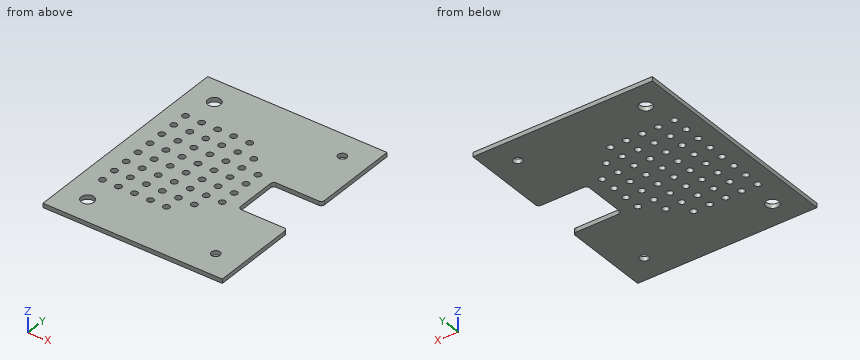
from build123d import *

# Parameters (mm, degrees)
F0_W     = 84
F0_H     = 104
F0_R     = 3
F0_R_2   = 2
F1_DEPTH = 2
F2_W     = 23
F2_H     = 22
F3_DEPTH = 2.001
F4_R     = 1.5
F5_R     = 1.5
F6_DEPTH = 2.001


with BuildPart() as f1:
    # F0 (on Top) → F1 (new body)
    with BuildSketch(Plane.XY):
        Rectangle(F0_W, F0_H)
        with Locations((-30, -40)):
            Circle(F0_R, mode=Mode.SUBTRACT)
        with Locations((30, -40)):
            Circle(F0_R_2, mode=Mode.SUBTRACT)
        with Locations((-30, 40)):
            Circle(F0_R, mode=Mode.SUBTRACT)
        with Locations((30, 40)):
            Circle(F0_R_2, mode=Mode.SUBTRACT)
    extrude(amount=F1_DEPTH)

    # F2 (on face) → F3 (cut, through all)
    with BuildSketch(Plane(origin=(0, 0, 0), x_dir=(1, 0, 0), z_dir=(0, 0, -1))):
        with Locations((30.5, 0)):
            Rectangle(F2_W, F2_H)
    extrude(amount=-F3_DEPTH, mode=Mode.SUBTRACT)

    # F4
    f4_edges = [f1.edges().sort_by_distance(p)[0] for p in [
        (19, 11, 1),
        (42, 11, 1),
        (19, -11, 1),
        (42, -11, 1),
    ]]
    fillet(f4_edges, radius=F4_R)

    # F5 (on face) → F6 (cut, through all)
    with BuildSketch(Plane.XY.offset(2)):
        with Locations((-33.25, -26.25)):
            Circle(F5_R)
        with Locations((-33.25, -18.75)):
            Circle(F5_R)
        with Locations((-33.25, -11.25)):
            Circle(F5_R)
        with Locations((-33.25, -3.75)):
            Circle(F5_R)
        with Locations((-25.75, -26.25)):
            Circle(F5_R)
        with Locations((-25.75, -18.75)):
            Circle(F5_R)
        with Locations((-25.75, -11.25)):
            Circle(F5_R)
        with Locations((-25.75, -3.75)):
            Circle(F5_R)
        with Locations((-18.25, -26.25)):
            Circle(F5_R)
        with Locations((-18.25, -18.75)):
            Circle(F5_R)
        with Locations((-18.25, -11.25)):
            Circle(F5_R)
        with Locations((-18.25, -3.75)):
            Circle(F5_R)
        with Locations((-10.75, -26.25)):
            Circle(F5_R)
        with Locations((-10.75, -18.75)):
            Circle(F5_R)
        with Locations((-10.75, -11.25)):
            Circle(F5_R)
        with Locations((-10.75, -3.75)):
            Circle(F5_R)
        with Locations((-3.25, -26.25)):
            Circle(F5_R)
        with Locations((-3.25, -18.75)):
            Circle(F5_R)
        with Locations((-3.25, -11.25)):
            Circle(F5_R)
        with Locations((-3.25, -3.75)):
            Circle(F5_R)
        with Locations((4.25, -18.75)):
            Circle(F5_R)
        with Locations((4.25, -11.25)):
            Circle(F5_R)
        with Locations((4.25, -3.75)):
            Circle(F5_R)
        with Locations((11.75, -11.25)):
            Circle(F5_R)
        with Locations((11.75, -3.75)):
            Circle(F5_R)
        with Locations((-33.25, 26.25)):
            Circle(F5_R)
        with Locations((-25.75, 26.25)):
            Circle(F5_R)
        with Locations((-25.75, 3.75)):
            Circle(F5_R)
        with Locations((-3.25, 3.75)):
            Circle(F5_R)
        with Locations((-10.75, 26.25)):
            Circle(F5_R)
        with Locations((-3.25, 26.25)):
            Circle(F5_R)
        with Locations((-33.25, 3.75)):
            Circle(F5_R)
        with Locations((-10.75, 3.75)):
            Circle(F5_R)
        with Locations((-33.25, 18.75)):
            Circle(F5_R)
        with Locations((-18.25, 3.75)):
            Circle(F5_R)
        with Locations((-18.25, 18.75)):
            Circle(F5_R)
        with Locations((-25.75, 11.25)):
            Circle(F5_R)
        with Locations((11.75, 11.25)):
            Circle(F5_R)
        with Locations((-25.75, 18.75)):
            Circle(F5_R)
        with Locations((-10.75, 18.75)):
            Circle(F5_R)
        with Locations((-33.25, 11.25)):
            Circle(F5_R)
        with Locations((-3.25, 18.75)):
            Circle(F5_R)
        with Locations((4.25, 18.75)):
            Circle(F5_R)
        with Locations((-10.75, 11.25)):
            Circle(F5_R)
        with Locations((11.75, 3.75)):
            Circle(F5_R)
        with Locations((-18.25, 26.25)):
            Circle(F5_R)
        with Locations((4.25, 3.75)):
            Circle(F5_R)
        with Locations((-3.25, 11.25)):
            Circle(F5_R)
        with Locations((4.25, 11.25)):
            Circle(F5_R)
        with Locations((-18.25, 11.25)):
            Circle(F5_R)
    extrude(amount=-F6_DEPTH, mode=Mode.SUBTRACT)


solid = f1.part
For this review, take the finished solid that the model builds, in its own axes (mm). Round coordinates to 2 decimals unless told otherwise and drop trailing zeros. Order: outer loops, then holes, each group sorted by start corner. A loop starts at its lowest first (then second) coordinate and runs counter-clockwise, first axis right, second up. Notation, with made-up numbers: (-31, 33) -> (0, 33) arc R9 cw to (0, 43) -> close; hole circle Ø10 at (14.25, 0.25). An arc over 180 degrees is marked (long way). Put each result on its own line as item: value.
Q1. For probe 1 along Y at (x, z) = (21, 0.75); probe 2 along Y at (x, z) = (-31.5, 0.8); probe 3 along Y at (x, z) = (-29.5, 1.3), list the stretches that pass through material, from the lowest coordinate up. Write a range as [from, to].
Check result:
probe 1: [-52, -11], [11, 52]
probe 2: [-52, -42.6], [-37.4, 37.4], [42.6, 52]
probe 3: [-52, -42.96], [-37.04, 37.04], [42.96, 52]
Q2. Add section D-D on x = 4.25. Write out the cut boundary in (y, z).
Check result:
outline: (-52, 0) -> (-20.25, 0) -> (-20.25, 2) -> (-52, 2) -> close; (-17.25, 0) -> (-12.75, 0) -> (-12.75, 2) -> (-17.25, 2) -> close; (-9.75, 0) -> (-5.25, 0) -> (-5.25, 2) -> (-9.75, 2) -> close; (-2.25, 0) -> (2.25, 0) -> (2.25, 2) -> (-2.25, 2) -> close; (5.25, 0) -> (9.75, 0) -> (9.75, 2) -> (5.25, 2) -> close; (12.75, 0) -> (17.25, 0) -> (17.25, 2) -> (12.75, 2) -> close; (20.25, 0) -> (52, 0) -> (52, 2) -> (20.25, 2) -> close
Q3. Insertion check: pin 1 Ø5 at (x, y) = (-25.75, 18.75) entering from +Z. The pin has a flat end and moves straight along its axis. Give the tip position at first contact, or say it passes through.
Check result:
pin 1: z = 2
Q4. Add section B-B on x = 25.5. Write out the cut boundary in (y, z), plus the area to 3 significant figures.
Check result:
outline: (-52, 0) -> (-11, 0) -> (-11, 2) -> (-52, 2) -> close; (11, 0) -> (52, 0) -> (52, 2) -> (11, 2) -> close
area: 164 mm2
Q5. Add section C-C on y = -3.75. State how many separate pieces and enclosed holes the cut face has, plus the area to 3 significant figures.
Check result:
separate pieces: 8
enclosed holes: 0
area: 80.0 mm2
Q6. Add section A-A on y = -40. Write out the cut boundary in (x, z).
Check result:
outline: (-42, 0) -> (-33, 0) -> (-33, 2) -> (-42, 2) -> close; (-27, 0) -> (28, 0) -> (28, 2) -> (-27, 2) -> close; (32, 0) -> (42, 0) -> (42, 2) -> (32, 2) -> close
